Can you work these out from the model? Positions are in its coordinate system, mm. Give positions to 0.01 mm unless a question says otherwise; leave off trailing zeros. Write each loop counter-clockwise with the first axis right and the second up, starting at its lowest first coordinate (ties: lowest second). Pieces come first, ordered by that corner, then holes.
1. Suppose I cut it at D-D (x = 35.5). Please give me the cut outline in (y, z).
2. Suppose I cut it at A-A (y = 21.5). Please give me the cut outline in (x, z), and give its area (3 significant figures).
3. Suppose I cut it at B-B (x = 0). Please give me the cut outline in (y, z).
4. If I drill on probe 1 along X at (y, z) = (45, 3.2); probe 2 along Y at (x, z) = (1, 3.3); probe 3 along Y at (x, z) = (12.5, 4.6), over which ranges is the centre line in solid material (lowest first)?
5. I'm going to push flat-ended pins straight in: pin 1 (4.5 mm diameter, centred on x = 14, y = 16.68, fed in from +Z); pin 2 (1.7 mm diameter, centred on x = 14, y = 44.68, fed in from +Z); pin 3 (2.5 mm diameter, centred on y = 33.5, z = 2.5, fed in from +X); pin 4 (1.5 mm diameter, centred on x = -0.5, z = 1.5, fed in from +Y). Where does each tip first touch, or does it pass through?
6. Suppose I cut it at C-C (x = -14). Please give me the cut outline in (y, z), and give its area (3 significant figures).
7. Thinking about a two-plate mould opening in Y: for faces 1 (the flat face through (1, -12.318, 2)), 2 (the cylindrical face through (-21.5, 9.2, 2.5)), 3 (the flat face through (8, 28, 5)), 4 (the cylindrical face through (0.88, 67.673, 2.535)), which applies, pulls with the +Y half, pulls with the -Y half, needs draft (parallel to the pull), parting line crosses it, or undercut?
Autodesk Inventor part; units mm, degrees
ref_plane "YZ Plane" through (0, 0, 0) normal (1, 0, 0) x (0, 1, 0)
ref_plane "XZ Plane" through (0, 0, 0) normal (0, 1, 0) x (-1, 0, 0)
ref_plane "XY Plane" through (0, 0, 0) normal (0, 0, 1) x (1, 0, 0)
sketch "スケッチ1" plane through (0, 0, 0) normal (0, 0, 1) x (1, 0, 0)
  line L0 (-40, 67.6823) -> (40, 67.6823)
  line L1 (40, 67.6823) -> (40, -12.3177)
  line L2 (40, -12.3177) -> (-40, -12.3177)
  line L3 (-40, -12.3177) -> (-40, 67.6823)
  point P0 (0, 0)
  dimension "d0" = 80
  dimension "d1" = 40
  dimension "d2" = 80
extrude "押し出し1" add sketch "スケッチ1" along normal blind 5
sketch "スケッチ5" plane through (0, 0, 5) normal (0, 0, 1) x (1, 0, 0)
  line L0 (-40, -7.3177) -> (40, -7.3177)
  line L1 (40, 67.6823) -> (40, -12.3177)
  line L2 (-40, 67.6823) -> (40, 67.6823)
  line L3 (-40, -12.3177) -> (-40, 67.6823)
  arc A0 (40, 27.6823) -> (-40, 27.6823) centre (0, 27.6823) ccw
  point P0 (0, 0)
  dimension "d21" = 40
  dimension "d22" = 40
  dimension "d23" = 80
extrude "押し出し4" cut sketch "スケッチ5" against normal through all contours L3 L2 A0 | A0 L2 L1
sketch "スケッチ6" plane through (0, 0, 5) normal (0, 0, 1) x (1, 0, 0)
  arc A0 (40, 27.6823) -> (-40, 27.6823) centre (0, 27.6823) ccw
  point P0 (0, 0)
hole "Hole2" at (0, 27.6823, 5) direction (0, 0, -1) diameter 8 end through all
sketch "スケッチ8" plane through (0, 0, 5) normal (0, 0, 1) x (1, 0, 0)
  circle A0 centre (0, 27.6823) radius 4
  line L0 (-20, 10.6823) -> (20, 10.6823)
  line L1 (20, 10.6823) -> (20, 7.6823)
  line L2 (20, 7.6823) -> (-20, 7.6823)
  line L3 (-20, 7.6823) -> (-20, 10.6823)
  circle A1 centre (-20, 9.1823) radius 1.5
  circle A2 centre (20, 9.1823) radius 1.5
  line L4 (40, -12.3177) -> (-40, -12.3177)
  line L5 (-20, 53.6823) -> (20, 53.6823)
  line L6 (20, 53.6823) -> (20, 50.6823)
  line L7 (20, 50.6823) -> (-20, 50.6823)
  line L8 (-20, 50.6823) -> (-20, 53.6823)
  circle A3 centre (-20, 52.1823) radius 1.5
  circle A4 centre (20, 52.1823) radius 1.5
  point P0 (0, 0)
  dimension "d54" = 3
  dimension "d55" = 20
  dimension "d56" = 40
  dimension "d65" = 20
  dimension "d87" = 40
  dimension "d88" = 20
  dimension "d89" = 3
  dimension "d91" = 40
extrude "押し出し5" cut sketch "スケッチ8" against normal through all contours A1 L3 | L0 A2 L2 A1 | L3 A1 | A2 L1 | L1 A2 | A3 L8 | L5 A4 L7 A3 | L8 A3 | A4 L6 | L6 A4
sketch "スケッチ9" plane through (0, 0, 5) normal (0, 0, 1) x (1, 0, 0)
  line L0 (-40, -12.3177) -> (-40, 27.6823)
  line L1 (40, -12.3177) -> (-40, -12.3177)
  line L2 (40, 27.6823) -> (40, -12.3177)
  line L3 (-30, -7.2177) -> (30, -7.2177)
  line L4 (30, -7.2177) -> (30, -10.2177)
  line L5 (30, -10.2177) -> (-30, -10.2177)
  line L6 (-30, -10.2177) -> (-30, -7.2177)
  circle A0 centre (-30, -8.7177) radius 1.5
  circle A1 centre (30, -8.7177) radius 1.5
  point P0 (0, 0)
  dimension "d59" = 3
  dimension "d60" = 10
  dimension "d61" = 10
  dimension "d62" = 5.1
extrude "押し出し6" cut sketch "スケッチ9" against normal through all
sketch "スケッチ11" plane through (0, 0, 5) normal (0, 0, 1) x (1, 0, 0)
  arc A0 (20, 50.6823) -> (20, 53.6823) centre (20, 52.1823) ccw
  line L0 (20, 50.6823) -> (-20, 50.6823)
  line L1 (-20, 10.6823) -> (20, 10.6823)
  arc A1 (-20, 10.6823) -> (-20, 7.6823) centre (-20, 9.1823) ccw
  point P0 (0, 0)
  point P1 (-14, 44.6823)
  point P2 (-14, 16.6823)
  point P3 (14, 16.6823)
  point P4 (14, 44.6823)
  dimension "d92" = 6
  dimension "d93" = 6
  dimension "d94" = 6
  dimension "d95" = 6
  dimension "d96" = 6
  dimension "d97" = 6
  dimension "d98" = 6
  dimension "d99" = 6
hole "Hole5" at (-14, 44.6823, 5) at (-14, 16.6823, 5) at (14, 16.6823, 5) at (14, 44.6823, 5) direction (0, 0, -1) diameter 2.8 depth 8 tip angle 118
sketch "スケッチ12" plane through (0, 0, 5) normal (0, 0, 1) x (1, 0, 0)
  circle A0 centre (0, 27.6823) radius 4
  line L0 (-4, 42.1823) -> (4, 42.1823)
  line L1 (4, 42.1823) -> (4, 19.1823)
  line L2 (4, 19.1823) -> (-4, 19.1823)
  line L3 (-4, 19.1823) -> (-4, 42.1823)
  circle A1 centre (0, 42.1823) radius 4
  circle A2 centre (0, 19.1823) radius 4
  circle A3 centre (14, 16.6823) radius 1.4
  circle A4 centre (-14, 44.6823) radius 1.4
  point P0 (0, 0)
  dimension "d109" = 2.5
  dimension "d110" = 2.5
extrude "押し出し7" cut sketch "スケッチ12" against normal blind 10 contours L1 A2 L3 A0 | A0 L3 A1 L1 | A1 L0 | L0 A1 | A2 L2 | L2 A2
equation "\"d2\" = d0"
equation "\"d55\" = 0.5 * d56"
equation "\"d87\" = d56"
equation "\"d88\" = d55"
equation "\"d89\" = d54"
equation "\"d61\" = d60"
equation "\"d110\" = d109"
properties part number "JointB1"
Checks:
1. outline: (-12.32, 0) - (46.11, 0) - (46.11, 5) - (-12.32, 5) - close
2. outline: (-40, 0) - (-4, 0) - (-4, 5) - (-40, 5) - close; (4, 0) - (40, 0) - (40, 5) - (4, 5) - close
2. area: 360 mm2
3. outline: (-12.32, 0) - (-10.22, 0) - (-10.22, 5) - (-12.32, 5) - close; (-7.22, 0) - (7.68, 0) - (7.68, 5) - (-7.22, 5) - close; (10.68, 0) - (15.18, 0) - (15.18, 5) - (10.68, 5) - close; (46.18, 0) - (50.68, 0) - (50.68, 5) - (46.18, 5) - close; (53.68, 0) - (67.68, 0) - (67.68, 5) - (53.68, 5) - close
4. probe 1: x = -36.06 to -15.36, -12.64 to -2.84, 2.84 to 12.64, 15.36 to 36.06
4. probe 2: y = -12.32 to -10.22, -7.22 to 7.68, 10.68 to 15.31, 46.06 to 50.68, 53.68 to 67.67
4. probe 3: y = -12.32 to -10.22, -7.22 to 7.68, 10.68 to 50.68, 53.68 to 65.68
5. pin 1: stops at z = 5
5. pin 2: passes through
5. pin 3: stops at x = 39.74
5. pin 4: stops at y = 67.68
6. outline: (-12.32, 0) - (-10.22, 0) - (-10.22, 5) - (-12.32, 5) - close; (-7.22, 0) - (7.68, 0) - (7.68, 5) - (-7.22, 5) - close; (10.68, 0) - (15.28, 0) - (15.28, 5) - (10.68, 5) - close; (18.08, 0) - (43.28, 0) - (43.28, 5) - (18.08, 5) - close; (46.08, 0) - (50.68, 0) - (50.68, 5) - (46.08, 5) - close; (53.68, 0) - (65.15, 0) - (65.15, 5) - (53.68, 5) - close
6. area: 314 mm2
7. face 1: pulls with the -Y half
7. face 2: undercut
7. face 3: needs draft
7. face 4: pulls with the +Y half
